Part model, mm, in its own coordinate system. Face numbers are marked on the shaded views. A direction names the side the tool comes from. Give positions to 0.01 mm unless a question says otherwise; leave off trailing zeros. Order: outer loops, then holes, each group sorted by start corner. A loop starts at its lowest first (then second) coordinate and runs counter-clockwise, first axis right, second up. Notation, with made-up numbers: (-20, 25.25) -> (2, 25.25) arc R24 ccw to (2, 43.25) -> close; hole circle Ø10 at (-10.5, -4.5). An arc over 180 degrees is marked (long way). Write item = value, one per line. Start each with the question number.
Item 1: Drill centre lines: line 1 along Z through (x, y) = (2, 53); line 2 along Y through (x, z) = (-3, 3.5) (3 decimals); line 3 along X through (y, z) = (31.5, -17). Where is each one in solid material? Low to high.
Item 2: Band-saw the part on A-A on y = 37. Write the cut outline in (x, z) (3 decimals), plus the area to 3 significant figures.
Item 3: Band-saw the part on C-C on x = 13.5. Write the cut outline in (y, z) (3 decimals).
Item 4: Band-saw the part on B-B on z = -11. Write the cut outline in (x, y) (1 decimal), plus the area to 3 significant figures.
Item 5: Flat gauge pins, fed straight in: P1, Ø3, axis at x = -21, y = 51, coming from the -Z side; P2, Ø3, axis at y = 34.5, z = 4.5, coming from the -X side; P3, Ø12, axis at x = -20, z = 4.5, coming from the +Y side. Where does each tip first touch, or does it go through?
Item 6: Tool access for the marked faces 5, 6 and 7: list every direction of +Z, -Z, +X, -X, +Y, -Y with a clear straight run to the whole face (end or side of a thin tool).
Item 7: Pull direction X, two halves, no side cores. Call the marked faces 1, 2, 3 and 4: +X half, -X half, draft (parallel to the pull), parting line (faces both ways), or undercut.
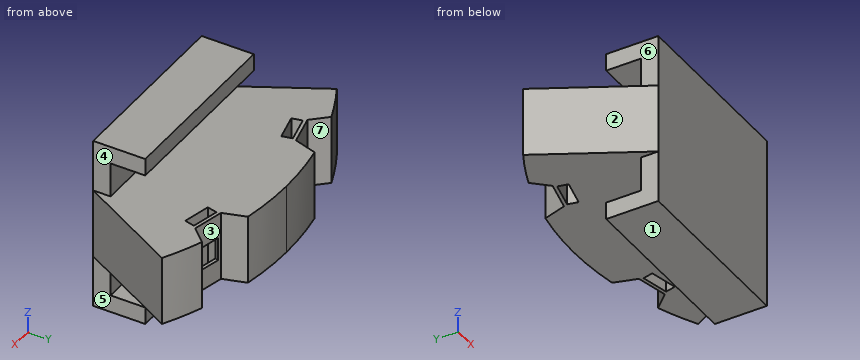
```python
from build123d import *

# Parameters (mm, degrees)
EXTRUSION1_DEPTH = 12.7
SKETCH2_R        = 0.0001
EXTRUSION2_DEPTH = 12.7
EXTRUSION3_REACH = 47.242
SKETCH3_W        = 3.81
SKETCH3_H        = 4.269275936
EXTRUSION4_REACH = 47.242
SKETCH4_W        = 3.81
SKETCH4_H        = 4.2672
SKETCH5_W        = 33.063140678
SKETCH5_H        = 3.175
EXTRUSION5_DEPTH = 9.525
SKETCH6_W        = 33.063140678
SKETCH6_H        = 3.175
EXTRUSION6_DEPTH = 6.35
SKETCH7_W        = 33.063140678
SKETCH7_H        = 3.175
EXTRUSION7_DEPTH = 9.525
SKETCH8_W        = 33.063140678
SKETCH8_H        = 3.175
EXTRUSION8_DEPTH = 6.35


with BuildPart() as part:
    # Sketch1 → Extrusion1 (new body)
    with BuildSketch(Plane.XY):
        with BuildLine():
            Line((-46.835285843, 30.48), (46.835285843, 30.48))
            ThreePointArc((46.835285843, 30.48), (26.639744744, 49.121262199), (0, 55.88))
            ThreePointArc((0, 55.88), (-26.639744744, 49.121262199), (-46.835285843, 30.48))
        make_face()
    extrude(amount=-EXTRUSION1_DEPTH)

    # Sketch2 → Extrusion2 (cut)
    with BuildSketch(Plane.XY):
        Polygon((-17.087387335, 49.474285222), (-11.424998154, 50.789978227), (-10.16, 54.948601438), (-13.629796213, 58.658980697), (-18.577977015, 57.50923866), (-20.056361604, 52.649117364), align=None)
        Polygon((18.577977015, 57.50923866), (13.629796213, 58.658980697), (10.16, 54.948601438), (11.424998154, 50.789978227), (17.087387335, 49.474285222), (20.056361604, 52.649117364), align=None)
        with Locations((-0.000275836, 0.000298823)):
            Circle(SKETCH2_R)
        with BuildLine():
            Line((-46.835285843, 30.48), (-0.000330381, 0.000215009))
            Line((-0.000330381, 0.000215009), (-26.641574626, 49.120269761))
            ThreePointArc((-26.641574626, 49.120269761), (-37.902205349, 41.060896601), (-46.835285843, 30.48))
        make_face()
        with Locations((0.000275836, 0.000298823)):
            Circle(SKETCH2_R)
        with BuildLine():
            Line((26.641574627, 49.120269761), (0.000187932, 0.0003465))
            Line((0.000187932, 0.0003465), (46.835285843, 30.48))
            ThreePointArc((46.835285843, 30.48), (37.902205349, 41.060896601), (26.641574627, 49.120269761))
        make_face()
        Polygon((11.207321789, 48.233301672), (16.155502591, 47.083559635), (16.586565391, 48.938738106), (11.638384589, 50.088480143), align=None)
        Polygon((-16.155412127, 47.083170305), (-11.207231325, 48.232912342), (-11.638384589, 50.088480143), (-16.586565391, 48.938738106), align=None)
    extrude(amount=-EXTRUSION2_DEPTH, mode=Mode.SUBTRACT)

    # Sketch3 → Extrusion3 (cut, up to next)
    with BuildSketch(Plane(origin=(-11.782102344, 50.707002743, 0), x_dir=(-0.9740513389582227, -0.22632717263663577, 0), z_dir=(-0.22632717263663577, 0.9740513389582227, 0)), mode=Mode.PRIVATE) as extrusion3_sk1:
        with Locations((2.54, -6.628362032)):
            Rectangle(SKETCH3_W, SKETCH3_H)
    extrusion3_tool1 = extrude(extrusion3_sk1.sketch, amount=-EXTRUSION3_REACH, mode=Mode.PRIVATE) & part.part
    add(extrusion3_tool1.solids().sort_by_distance((-14.256193, 50.132132, -6.628362))[0], mode=Mode.SUBTRACT)

    # Sketch4 → Extrusion4 (cut, up to next)
    with BuildSketch(Plane(origin=(11.782102344, 50.707002743, 0), x_dir=(-0.974051338958225, 0.22632717263662588, 0), z_dir=(0.2263271726366259, 0.9740513389582252, 0)), mode=Mode.PRIVATE) as extrusion4_sk1:
        with Locations((-2.173382579, -6.6294)):
            Rectangle(SKETCH4_W, SKETCH4_H)
    extrusion4_tool1 = extrude(extrusion4_sk1.sketch, amount=-EXTRUSION4_REACH, mode=Mode.PRIVATE) & part.part
    add(extrusion4_tool1.solids().sort_by_distance((13.899089, 50.215107, -6.6294))[0], mode=Mode.SUBTRACT)

    # Sketch5 → Extrusion5 (add)
    with BuildSketch(Plane(origin=(0, 0, -12.7), x_dir=(-1, 0, 0), z_dir=(0, 0, -1))):
        with Locations((0, 32.0675)):
            Rectangle(SKETCH5_W, SKETCH5_H)
    extrude(amount=EXTRUSION5_DEPTH)

    # Sketch6 → Extrusion6 (add)
    with BuildSketch(Plane(origin=(0, 33.655, 0), x_dir=(-1, 0, 0), z_dir=(0, 1, 0))):
        with Locations((0, -20.6375)):
            Rectangle(SKETCH6_W, SKETCH6_H)
    extrude(amount=EXTRUSION6_DEPTH)

    # Sketch7 → Extrusion7 (add)
    with BuildSketch(Plane.XY):
        with Locations((0, 32.0675)):
            Rectangle(SKETCH7_W, SKETCH7_H)
    extrude(amount=EXTRUSION7_DEPTH)

    # Sketch8 → Extrusion8 (add)
    with BuildSketch(Plane(origin=(0, 33.655, 0), x_dir=(-1, 0, 0), z_dir=(0, 1, 0))):
        with Locations((0, 7.9375)):
            Rectangle(SKETCH8_W, SKETCH8_H)
    extrude(amount=EXTRUSION8_DEPTH)


solid = part.part
```
Values found:
q1.line_1 = -12.7 to 0
q1.line_2 = 30.48 to 33.655
q1.line_3 = -16.53 to 16.53
q2.outline = (-20.068, -12.7) -> (20.068, -12.7) -> (20.068, 0) -> (-20.068, 0) -> close; (-16.532, -22.225) -> (16.532, -22.225) -> (16.532, -19.05) -> (-16.532, -19.05) -> close; (-16.532, 6.35) -> (16.532, 6.35) -> (16.532, 9.525) -> (-16.532, 9.525) -> close
q2.area = 720 mm^2
q3.outline = (30.48, -22.225) -> (40.005, -22.225) -> (40.005, -19.05) -> (33.655, -19.05) -> (33.655, -12.7) -> (47.701, -12.7) -> (47.701, 0) -> (33.655, 0) -> (33.655, 6.35) -> (40.005, 6.35) -> (40.005, 9.525) -> (30.48, 9.525) -> close; (49.656, -12.7) -> (50.308, -12.7) -> (50.308, -8.763) -> (49.656, -8.763) -> close; (49.656, -4.496) -> (50.308, -4.496) -> (50.308, 0) -> (49.656, 0) -> close
q4.outline = (-26.6, 49.1) -> (-16.5, 30.5) -> (16.5, 30.5) -> (26.6, 49.1) arc R55.9 ccw to (19.7, 52.3) -> (17.1, 49.5) -> (11.4, 50.8) -> (10.2, 54.9) arc R55.9 ccw to (-10.2, 54.9) -> (-11.4, 50.8) -> (-17.1, 49.5) -> (-19.7, 52.3) arc R55.9 ccw to start; hole (-16.6, 48.9) -> (-16.2, 47.1) -> (-11.2, 48.2) -> (-11.6, 50.1) -> close; hole (11.2, 48.2) -> (16.2, 47.1) -> (16.6, 48.9) -> (11.6, 50.1) -> close
q4.area = 970 mm^2
q5.P1 = -12.7
q5.P2 = -16.53
q5.P3 = 52.29
q6.face_5 = -Z, +X, +Y, -Y
q6.face_6 = +Z, -X, +Y, -Y
q6.face_7 = +Z, -Z, +Y
q7.face_1 = draft
q7.face_2 = -X half
q7.face_3 = undercut
q7.face_4 = +X half
